Geometry: final body of the model. Coordinates: model frame, mm. A direction names the side the tool comes from. Give positions to 0.01 mm unless a question says otherwise; leave off trailing zeros. Order: outer loops, then holes, each group sorted by start corner. A loop starts at its lowest first (then second) coordinate and runs counter-clockwise, first axis right, second up. Notation, with made-up numbers: (27.5, 28) - (36.5, 28) arc R10 ccw to (36.5, 38) - close; hole circle Ø6 at (36, 17.5). An arc over 180 degrees is marked (long way). Put each result on its own line as item: value. Start each with the question number.
1. Ray query, line 1 along Z through (x, y) = (-13.5, -2); line 2 along Y through (x, z) = (41, -4.75); line 3 along Y through (x, z) = (2, 2.75). Return the intervals inside material, ascending. Write a range as from..to.
2. First-contact query: P1, Ø5, axis at x = 4, y = -3, coming from the -Z side; P2, Ø6, axis at x = 21.5, z = 1.5, coming from the -Y side; P3, Ø3, axis at x = 14, z = 3.5, coming from the -Y side. Flat tips, straight axial feed; report the tip coordinate or a pass-through.
3. Section A-A on x = 22. Return the cut outline in (y, z), plus the area to 3 significant figures.
4. Section B-B on x = 3. Return the cut outline in (y, z), plus the area to 3 significant figures.
5. Set-up query: faces 1 (the conical face through (6.68, 2.2, 4.22)), 2 (the flat face through (46.12, 0, 0)). Return all of +Z, -Z, +X, -X, +Y, -Y with unobstructed straight access to the full face (end or side cutting, diameter ignored); none if empty.
from build123d import *

# Parameters (mm, degrees)
SCHNITT_LINEAR_START            = -5
SKIZZE2_R                       = 2.5
SCHNITT_LINEAR_AUSTRAGEN1_DEPTH = 5
SKIZZE3_R                       = 4
SCHNITT_LINEAR_AUSTRAGEN2_DEPTH = 5


with BuildPart() as part:
    # Skizze1 → Rotation1 (revolve)
    with BuildSketch(Plane.XY):
        Polygon((-38.880400098, 0), (-38.880400098, 2.5), (-33.880400098, 2.5), (-33.880400098, 4), (46.119599902, 5.5), (46.119599902, 4), (51.119599902, 4), (51.119599902, 0), align=None)
    revolve(axis=Axis((51.119599902, 0, 0), (-1, 0, 0)))

    # Skizze2 → Schnitt-Linear austragen1 (cut)
    with BuildSketch(Plane.ZY.offset(38.880400098).offset(SCHNITT_LINEAR_START)):
        Circle(SKIZZE2_R)
    extrude(amount=SCHNITT_LINEAR_AUSTRAGEN1_DEPTH, mode=Mode.SUBTRACT)

    # Skizze3 → Schnitt-Linear austragen2 (cut)
    with BuildSketch(Plane(origin=(51.119599902, 0, 0), x_dir=(0, 0, -1), z_dir=(1, 0, 0))):
        Circle(SKIZZE3_R)
    extrude(amount=-SCHNITT_LINEAR_AUSTRAGEN2_DEPTH, mode=Mode.SUBTRACT)


solid = part.part
Resolved:
1. line 1: -3.9..3.9
1. line 2: -2.58..2.58
1. line 3: -3.78..3.78
2. P1: z = -4.69
2. P2: y = -5.09
2. P3: y = -4.47
3. outline: circle Ø10.1 at (0, 0)
3. area: 80.0 mm^2
4. outline: circle Ø9.38 at (0, 0)
4. area: 69.1 mm^2
5. face 1: -X
5. face 2: +Z, -Z, +X, +Y, -Y
